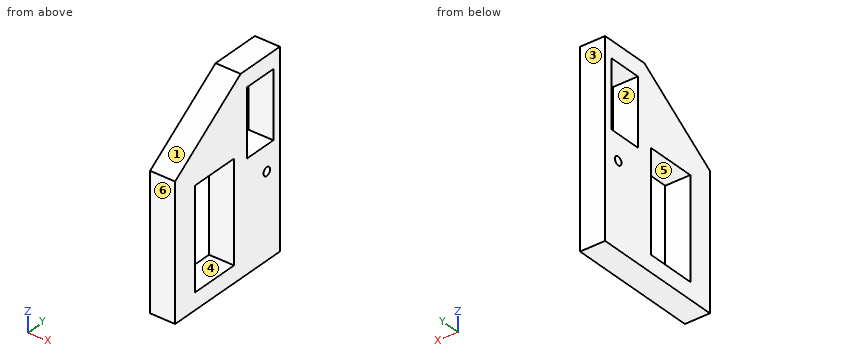
```python
from build123d import *

# Parameters (mm, degrees)
SKETCH1_W           = 40
SKETCH1_H           = 20
SKETCH1_W_2         = 60
SKETCH1_H_2         = 30
BOSS_EXTRUDE1_DEPTH = 15
SKETCH2_R           = 2.5
CUT_EXTRUDE1_DEPTH  = 15


with BuildPart() as part:
    # Sketch1 → Boss-Extrude1 (new body)
    with BuildSketch(Plane(origin=(0, 0, 0), x_dir=(0, 0, -1), z_dir=(1, 0, 0))):
        Polygon((-115, 50), (-80, 0), (0, 0), (0, 80), (-115, 80), align=None)
        with Locations((-85, 65)):
            Rectangle(SKETCH1_W, SKETCH1_H, mode=Mode.SUBTRACT)
        with Locations((-40, 30)):
            Rectangle(SKETCH1_W_2, SKETCH1_H_2, mode=Mode.SUBTRACT)
    extrude(amount=BOSS_EXTRUDE1_DEPTH)

    # Sketch2 → Cut-Extrude1 (cut)
    with BuildSketch(Plane(origin=(15, 0, 0), x_dir=(0, 0, -1), z_dir=(1, 0, 0))):
        with Locations((-50, 70)):
            Circle(SKETCH2_R)
    extrude(amount=-CUT_EXTRUDE1_DEPTH, mode=Mode.SUBTRACT)


solid = part.part
```
Work out the finished part from the listing and answer in its coordinate system (mm). Face numbers are marked on the shaded views. A direction names the side the tool comes from. Give positions to 0.01 mm unless a question says otherwise; leave off trailing zeros. Loops run counter-clockwise (first coordinate to the right, second up) from the corner with the lowest first, then second, coordinate; pieces in that order, holes last. Notation, with made-up numbers: (-6.75, 31) -> (21.25, 31) arc R27 ccw to (21.25, 55) -> close; hole circle Ø5 at (-6.75, -24). An arc over 180 degrees is marked (long way). One line per question, with ' | ' between items. Start each with the question number.
1) Section B-B, the plane x = 9.5 is taken. Determine the outline of the cut face in (y, z).
2) Straight lines are drawn through the part: L1, parallel to Y at x = 11.5, z = 50; L2, parallel to Y at x = 11, z = 43.5; L3, parallel to Z at x = 6.5, y = 69. For each, find the intervals that lie inside material, in ascending order.
3) Section D-D, the plane y = 70 is taken. Determine the outline of the cut face in (x, z).
4) Section A-A, the plane y = 27.5 is taken. Determine the outline of the cut face in (x, z), then the cut area to 3 significant figures.
5) This flat-tipped pin is pushed along its axis until it touches: pin 1 (4.5 mm diameter, centred on x = 10.5, y = 31.5, fed in from +Z) (3 decimals). Where does it stop, or does it pass through?
6) Section C-C, the plane z = 33.5 is taken. Determine the outline of the cut face in (x, y), then the cut area to 3 significant figures.
7) Determine the mould class of the marked faces 1, 2, 3 and 4 for opening direction Z: +Z half, -Z half, draft (parallel to the pull), parting line (faces both ways), or undercut.
8) For the marked faces 5 and 6, determine the directions among +Z, -Z, +X, -X, +Y, -Y from which every point of the face is accessible in a straight line to the end or side of a thin tool.
Resolved:
1) outline: (0, 0) -> (80, 0) -> (80, 115) -> (50, 115) -> (0, 80) -> close; hole (15, 10) -> (45, 10) -> (45, 70) -> (15, 70) -> close; hole (55, 65) -> (75, 65) -> (75, 105) -> (55, 105) -> close; hole circle Ø5 at (70, 50)
2) L1: 0 to 15, 45 to 67.5, 72.5 to 80 | L2: 0 to 15, 45 to 80 | L3: 0 to 47.71, 52.29 to 65, 105 to 115
3) outline: (0, 0) -> (15, 0) -> (15, 47.5) -> (0, 47.5) -> close; (0, 52.5) -> (15, 52.5) -> (15, 65) -> (0, 65) -> close; (0, 105) -> (15, 105) -> (15, 115) -> (0, 115) -> close
4) outline: (0, 0) -> (15, 0) -> (15, 10) -> (0, 10) -> close; (0, 70) -> (15, 70) -> (15, 99.25) -> (0, 99.25) -> close | area: 589 mm2
5) pin 1: z = 103.625
6) outline: (0, 0) -> (15, 0) -> (15, 15) -> (0, 15) -> close; (0, 45) -> (15, 45) -> (15, 80) -> (0, 80) -> close | area: 750 mm2
7) face 1: +Z half | face 2: undercut | face 3: draft | face 4: undercut
8) face 5: +X, -X | face 6: +Z, -Z, +X, -X, -Y
